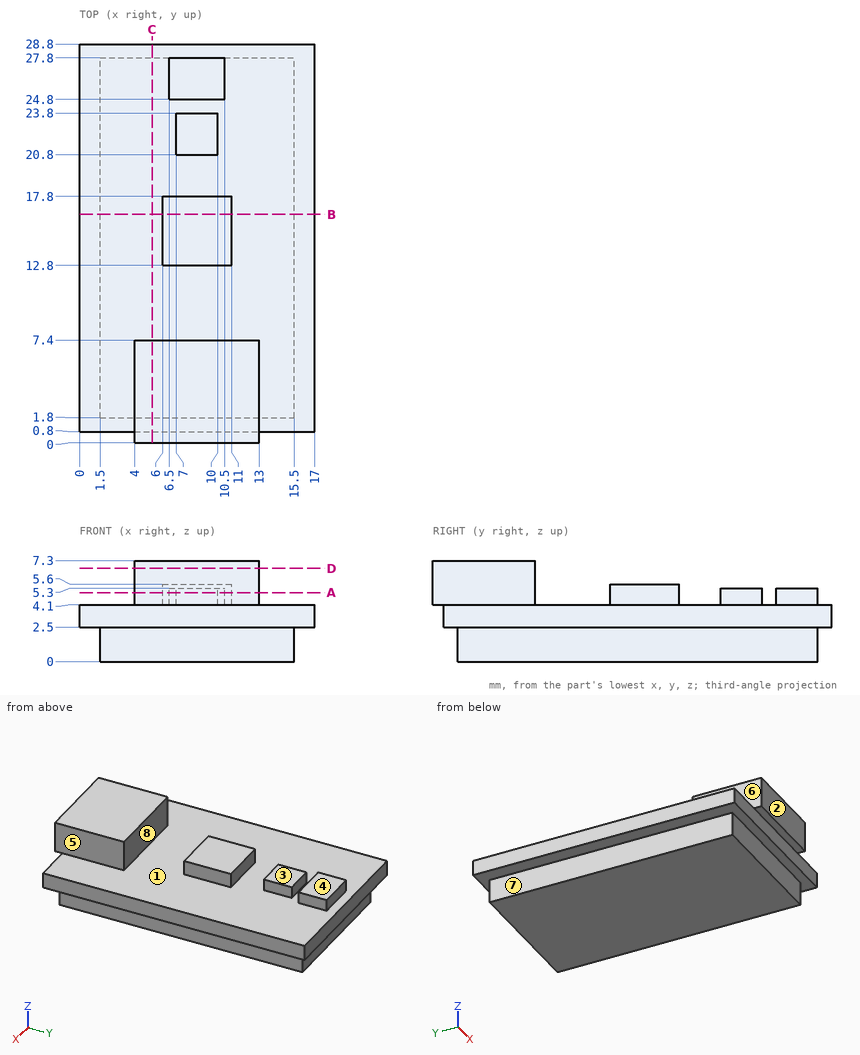
Geometry: see drawing. Coordinates: mm, zero at the bounding-box minimum. A direction names the side the tool comes from. Coordinates: 2 decimals unless noted, no trailing zeros. Order: outer loops, then holes, each group sorted by start corner. A loop starts at its lowest first (then second) coordinate and runs counter-clockwise, first axis right, second up. Notation, with made-up numbers: (88.25, 65.5) - (92.25, 65.5) arc R12 cw to (92.25, 78.5) - close; hole circle Ø8 at (29.25, 69). An arc over 180 degrees is marked (long way). Write each question's results on one line, items separated by ' | '.
(1) Line query: line 1 (X direction, y = 16, z = 4.25); line 2 (Y direction, x = 3.25, z = 3.25); line 3 (Y direction, x = 9, z = 1). Output: solid intervals per line, ascending. Write a range as [from, to].
Values found:
line 1: x = [6, 11] | line 2: y = [0.8, 28.8] | line 3: y = [1.8, 27.8]
(2) Section query C-C, the plane x = 5.25. Return the cut outline in (y, z), plus the area to 3 significant figures.
Values found:
outline: (0, 4.1) - (0.8, 4.1) - (0.8, 2.5) - (1.8, 2.5) - (1.8, 0) - (27.8, 0) - (27.8, 2.5) - (28.8, 2.5) - (28.8, 4.1) - (7.4, 4.1) - (7.4, 7.3) - (0, 7.3) - close | area: 133 mm²
(3) First-contact query: pin 1 Ø1.6 at (y, z) = (5, 5.5) entering from +X; pin 2 Ø1 at (y, z) = (3.5, 6) entering from -X; pin 3 Ø4 at (x, y) = (12.5, 14.5) entering from -Z; pin 4 Ø0.8 at (x, z) = (5.5, 1.5) entering from -Y. Flat tips, straight axial feed; report the tip coordinate or a pass-through.
Values found:
pin 1: stops at x = 13 | pin 2: stops at x = 4 | pin 3: stops at z = 0 | pin 4: stops at y = 1.8
(4) Section query B-B, the plane y = 16.5. Return the cut outline in (x, z).
Values found:
outline: (0, 2.5) - (1.5, 2.5) - (1.5, 0) - (15.5, 0) - (15.5, 2.5) - (17, 2.5) - (17, 4.1) - (11, 4.1) - (11, 5.6) - (6, 5.6) - (6, 4.1) - (0, 4.1) - close
(5) Section query D-D, the plane z = 6.75. Return the cut outline in (x, y).
Values found:
outline: (4, 0) - (13, 0) - (13, 7.4) - (4, 7.4) - close
(6) Set-up query: the marked faces 4, 5, 6, 7 and 8. Return all of +Z, -Z, +X, -X, +Y, -Y with unobstructed straight access to the full face (end or side cutting, diameter ignored); none if empty.
Values found:
face 4: +Z, +X, -X, +Y | face 5: +Z, +X, +Y, -Y | face 6: +Z, -X, +Y, -Y | face 7: -Z, -X, +Y, -Y | face 8: +Z, +X, -X
(7) Section query A-A, the plane z = 5. Return the cut outline in (x, y), plus the area to 3 significant figures.
Values found:
outline: (4, 0) - (13, 0) - (13, 7.4) - (4, 7.4) - close; (6, 12.8) - (11, 12.8) - (11, 17.8) - (6, 17.8) - close; (6.5, 24.8) - (10.5, 24.8) - (10.5, 27.8) - (6.5, 27.8) - close; (7, 20.8) - (10, 20.8) - (10, 23.8) - (7, 23.8) - close | area: 113 mm²
(8) Mould query, pull axis Y, two halves, no side actions, for the marked faces 1, 2 and 3. Classes: +Y half, -Y half, draft (parallel to the pull), parting line (faces both ways), or undercut.
Values found:
face 1: undercut | face 2: -Y half | face 3: draft
